Could you check a few things on this drawing? It's one solid part, dimensions in mm from its lowest x, y, z. Give positions to 0.01 mm unless a question says otherwise; leave off trailing zeros. Loops run counter-clockwise (first coordinate to the right, second up) from the corner with the lowest first, then second, coordinate; pieces in that order, holes last.
1. Imagine slicing it at B-B (z = 3.5). List the corners of the cut face in (x, y) for me.
2. Thinking about a two-plate mould opening in Y: for the marked faces 1 and 2, which applies, +Y half, -Y half, draft (parallel to the pull), parting line (faces both ways), or undercut?
3. Imagine slicing it at A-A (x = 13). List the corners of the cut face in (y, z) for me.
4. I need wall thicknesses on line 1 along Y through (x, z) = (14.5, 4.1); line 2 along X through (y, z) = (15.5, 4); line 3 along Z through (x, y) = (5, 11.5). Which ranges of each line are inside material? Lowest first, please.
5. Imagine slicing it at C-C (y = 9). List the corners of the cut face in (x, z) for me, plus the area to 3 significant figures.
6. Imagine slicing it at D-D (x = 47.5). List the corners of the cut face in (y, z) for me.
7. For P1, Ø10, axis at x = 13, y = 12.5, coming from the +Z side; P2, Ø1.3, axis at x = 34.5, z = 4, coming from the -Y side; P3, Ø2, axis at x = 16.5, z = 4, coming from the +Y side, each with a flat end and sliding along its axis, tell me the tip position at first contact or that it passes through.
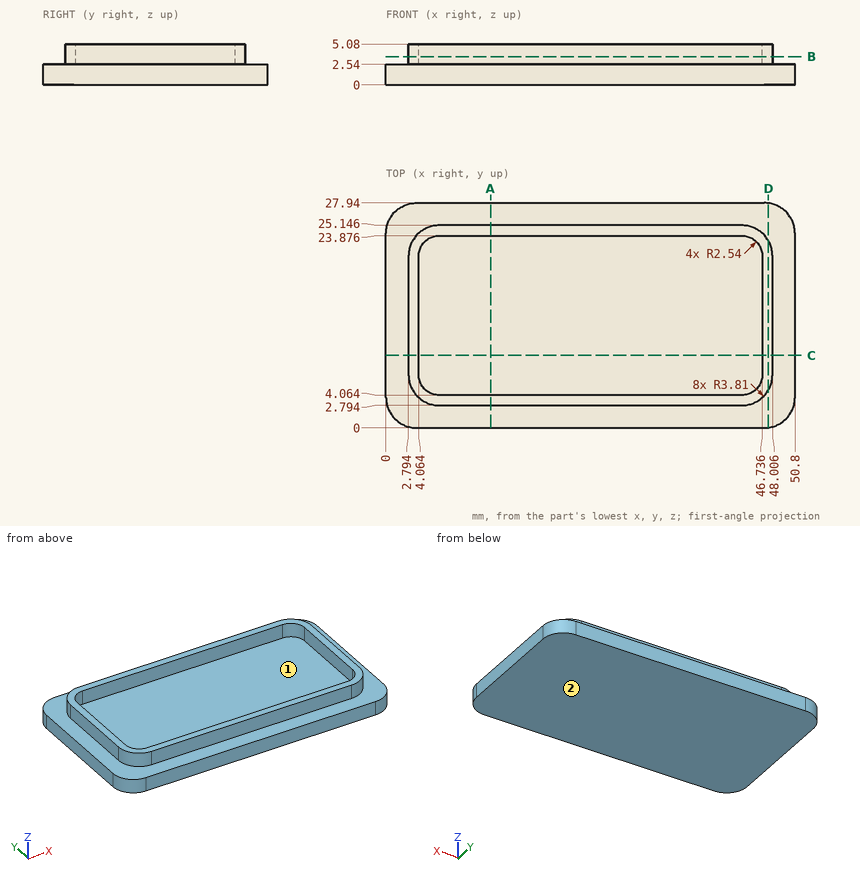
Derived:
1. outline: (2.79, 6.6) arc R3.81 ccw to (6.6, 2.79) - (44.2, 2.79) arc R3.81 ccw to (48.01, 6.6) - (48.01, 21.34) arc R3.81 ccw to (44.2, 25.15) - (6.6, 25.15) arc R3.81 ccw to (2.79, 21.34) - close; hole (4.06, 6.6) arc R2.54 ccw to (6.6, 4.06) - (44.2, 4.06) arc R2.54 ccw to (46.74, 6.6) - (46.74, 21.34) arc R2.54 ccw to (44.2, 23.88) - (6.6, 23.88) arc R2.54 ccw to (4.06, 21.34) - close
2. face 1: undercut
2. face 2: draft
3. outline: (0, 0) - (27.94, 0) - (27.94, 2.54) - (25.15, 2.54) - (25.15, 5.08) - (23.88, 5.08) - (23.88, 2.54) - (4.06, 2.54) - (4.06, 5.08) - (2.79, 5.08) - (2.79, 2.54) - (0, 2.54) - close
4. line 1: y = 2.79 to 4.06, 23.88 to 25.15
4. line 2: x = 2.79 to 4.06, 46.74 to 48.01
4. line 3: z = 0 to 2.54
5. outline: (0, 0) - (50.8, 0) - (50.8, 2.54) - (48.01, 2.54) - (48.01, 5.08) - (46.74, 5.08) - (46.74, 2.54) - (4.06, 2.54) - (4.06, 5.08) - (2.79, 5.08) - (2.79, 2.54) - (0, 2.54) - close
5. area: 135 mm2
6. outline: (0.03, 0) - (27.91, 0) - (27.91, 2.54) - (23.23, 2.54) - (23.23, 5.08) - (4.71, 5.08) - (4.71, 2.54) - (0.03, 2.54) - close
7. P1: stops at z = 2.54
7. P2: stops at y = 2.79
7. P3: stops at y = 25.15
